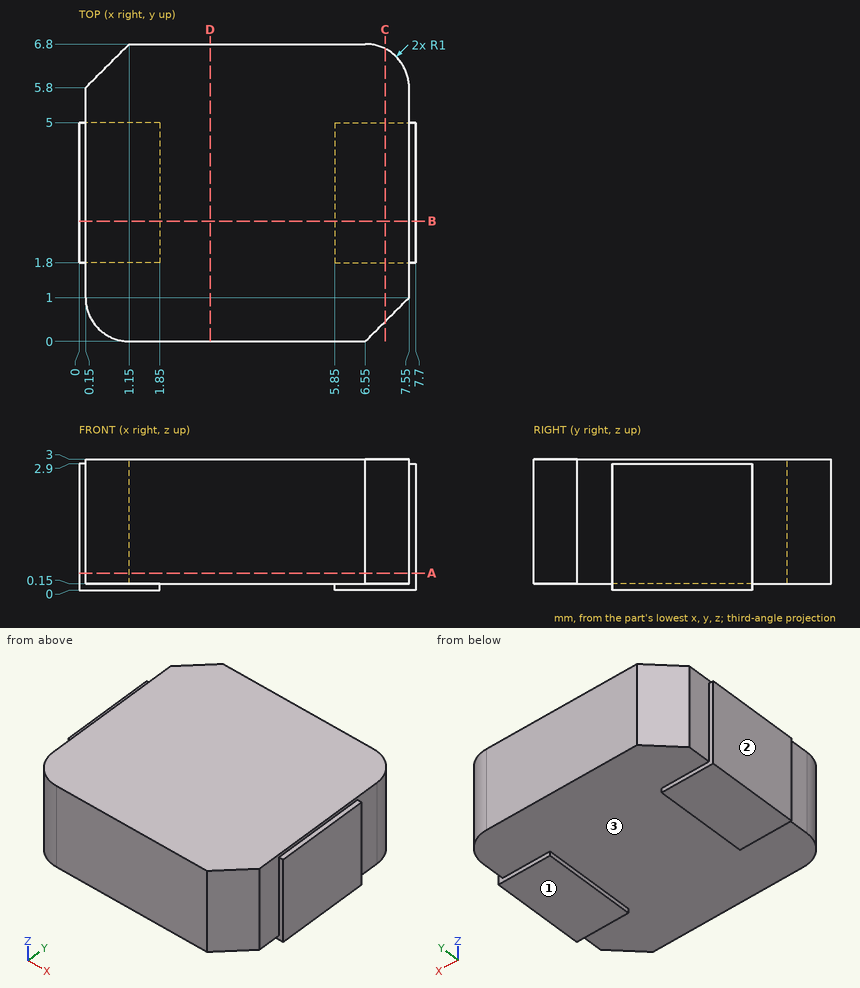
Study the drawing (mm; zero at the part's minimum x, y, z) and answer. Coordinates: 2 decimals unless noted, no trailing zeros. Order: outer loops, then holes, each group sorted by start corner. A loop starts at its lowest first (then second) coordinate and runs counter-clockwise, first axis right, second up. Notation, with made-up numbers: M -18.75,73.25 L 23.25,73.25 A23 cw 23.25,108.25 Z; hole C -15,14.25 d7. An arc over 180 degrees is marked long. Use CSV: the item, a comma, the result in double quotes.
Q1. Section C-C (x = 7) is taken. Determine the outline of the cut face in (y, z), then the cut area to 3 significant figures.
Here are the results:
outline,"M 0.45,0.15 L 1.8,0.15 L 1.8,0 L 5,0 L 5,0.15 L 6.69,0.15 L 6.69,3 L 0.45,3 Z"
area,"18.3 mm2"
Q2. Straight lines are drawn through the part: L1, parallel to Z at x = 5, y = 5.5; L2, parallel to X at y = 1.25, z = 0.4; L3, parallel to Y at x = 7, z = 1.05. For each, find the intervals that lie inside material, in ascending order.
Here are the results:
L1,"0.15 to 3"
L2,"0.15 to 7.55"
L3,"0.45 to 6.69"
Q3. Section A-A (z = 0.4) is taken. Determine the outline of the cut face in (x, y), then the cut area to 3 significant figures.
Here are the results:
outline,"M 0,1.8 L 0.15,1.8 L 0.15,1 A1 ccw 1.15,0 L 6.55,0 L 7.55,1 L 7.55,1.8 L 7.7,1.8 L 7.7,5 L 7.55,5 L 7.55,5.8 A1 ccw 6.55,6.8 L 1.15,6.8 L 0.15,5.8 L 0.15,5 L 0,5 Z"
area,"49.9 mm2"
Q4. Section D-D (x = 3) is taken. Determine the outline of the cut face in (y, z).
Here are the results:
outline,"M 0,0.15 L 6.8,0.15 L 6.8,3 L 0,3 Z"
Q5. Section B-B (y = 2.75) is taken. Determine the outline of the cut face in (x, z).
Here are the results:
outline,"M 0,0 L 1.85,0 L 1.85,0.15 L 5.85,0.15 L 5.85,0 L 7.7,0 L 7.7,2.9 L 7.55,2.9 L 7.55,3 L 0.15,3 L 0.15,2.9 L 0,2.9 Z"
Q6. Determine the mould class of the marked faces 1, 2 and 3 for opening direction X: pulls with the +X half, pulls with the -X half, needs draft (parallel to the pull), parting line crosses it, or undercut.
Here are the results:
face 1,"needs draft"
face 2,"pulls with the -X half"
face 3,"undercut"
